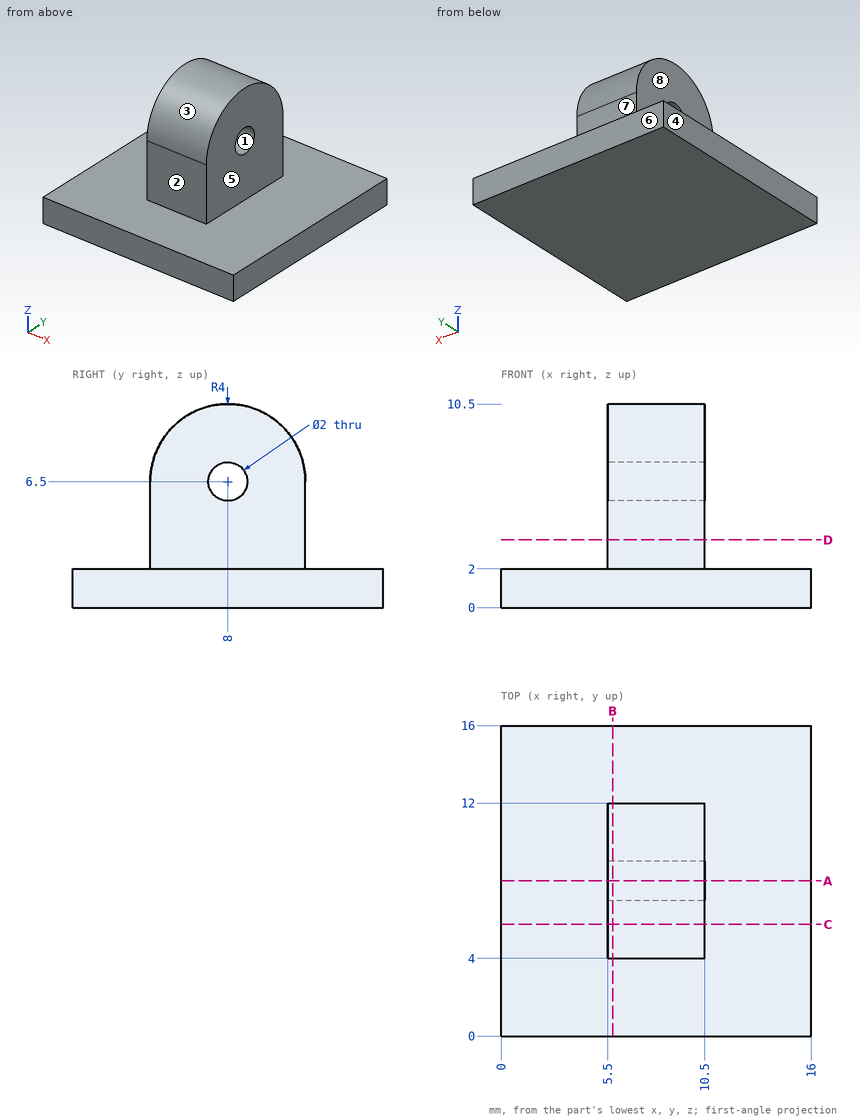
Geometry check sheet. Reference: drawing and pictorial views, mm from the part's lowest x, y, z. A direction names the side the tool comes from. Round coordinates to 2 decimals unless told otherwise and drop trailing zeros. Loops run counter-clockwise (first coordinate to the right, second up) from the corner with the lowest first, then second, coordinate; pieces in that order, holes last.
1. Sectioned sample at D-D on z = 3.5. Record the boundary of the cut face in (x, y), and give its area (3 significant figures).
2. Mould release check, pull along Z, two halves, no side actions. Record for the marked faces 1, 2 and 3: released by +Z, released by -Z, zero draft, split by the parting line, or undercut.
3. Set-up check for the marked faces 4, 5, 6, 7 and 8: record each of +Z, -Z, +X, -X, +Y, -Y from which the full face is reachable in a straight line by a thin tool's end or side.
4. Sectioned sample at C-C on y = 5.75. Record the boundary of the cut face in (x, z), and give its area (3 significant figures).
5. Gauge pin test, flat ends, axial feed: pin 1 Ø1 at (x, y) = (5.5, 3.5) entering from -Z; pin 2 Ø8 at (x, y) = (13.5, 3.5) entering from +Z; pin 3 Ø5 at (x, z) = (8.5, 5.5) entering from -Y; pin 4 Ø2.5 at (y, z) = (8, 6.5) entering from +X. Record the tip position at first contact, or that the pin passes through.
6. Sectioned sample at A-A on y = 8. Record the boundary of the cut face in (x, z), and give its area (3 significant figures).
7. Sectioned sample at B-B on x = 5.75. Record the boundary of the cut face in (y, z), and give its area (3 significant figures).
8. Scan lines: probe 1 along Z at (x, y) = (8.5, 8); probe 2 along X at (y, z) = (9.75, 8); probe 3 along Z at (x, y) = (12, 10). Record each from-to range of solid material in increasing order.
Recorded:
1. outline: (5.5, 4) - (10.5, 4) - (10.5, 12) - (5.5, 12) - close
1. area: 40.0 mm2
2. face 1: undercut
2. face 2: zero draft
2. face 3: released by +Z
3. face 4: +Z, -Z, -X, +Y, -Y
3. face 5: +Z, +X, +Y, -Y
3. face 6: +Z, -Z, +X, -X, +Y
3. face 7: +Z, +X, -X, +Y
3. face 8: +Z, -X, +Y, -Y
4. outline: (0, 0) - (16, 0) - (16, 2) - (10.5, 2) - (10.5, 9.81) - (5.5, 9.81) - (5.5, 2) - (0, 2) - close
4. area: 71.0 mm2
5. pin 1: stops at z = 0
5. pin 2: stops at z = 10.04
5. pin 3: stops at y = 4
5. pin 4: stops at x = 10.5
6. outline: (0, 0) - (16, 0) - (16, 2) - (10.5, 2) - (10.5, 5.5) - (5.5, 5.5) - (5.5, 2) - (0, 2) - close; (5.5, 7.5) - (10.5, 7.5) - (10.5, 10.5) - (5.5, 10.5) - close
6. area: 64.5 mm2
7. outline: (0, 0) - (16, 0) - (16, 2) - (12, 2) - (12, 6.5) arc R4 ccw to (4, 6.5) - (4, 2) - (0, 2) - close; hole circle Ø2 at (8, 6.5)
7. area: 90.0 mm2
8. probe 1: z = 0 to 5.5, 7.5 to 10.5
8. probe 2: x = 5.5 to 10.5
8. probe 3: z = 0 to 2
